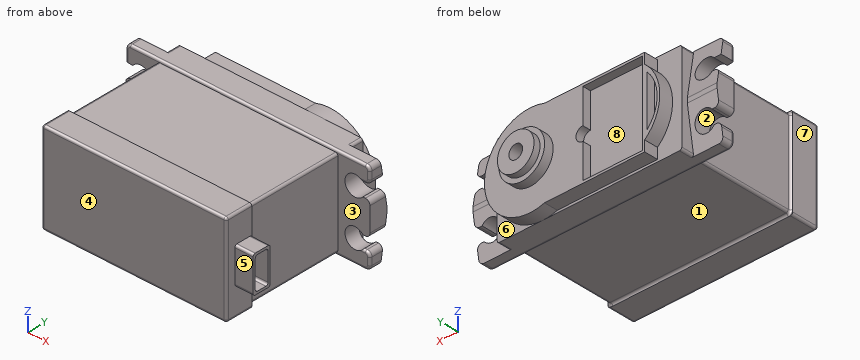
from build123d import *

# Parameters (mm, degrees)
SKETCH_2_W               = 40.3
SKETCH_2_H               = 32
EXTRUDE_1_DEPTH          = 20
SKETCH_3_W               = 20
SKETCH_3_H               = 4
EXTRUDE_2_DEPTH          = 6.5
CUT_EXTRUDE_4_DEPTH      = 6.5
SKETCH_4_W               = 20
SKETCH_4_H               = 4
EXTRUDE_3_DEPTH          = 6.5
CUT_EXTRUDE_5_DEPTH      = 6.5
CUT_EXTRUDE_6_DEPTH      = 43.284026865
CUT_EXTRUDE_6_DEPTH_BACK = 1.5
SKETCH_7_W               = 8
SKETCH_7_H               = 4
SKETCH_7_W_2             = 7
SKETCH_7_H_2             = 3
EXTRUDE_4_DEPTH          = 4
EXTRUDE_5_DEPTH          = 3
SKETCH_9_R               = 5
EXTRUDE_6_DEPTH          = 2
SKETCH_10_R              = 4
EXTRUDE_7_DEPTH          = 1.4
SKETCH_11_R              = 1.5
CUT_EXTRUDE_3_DEPTH      = 6.4
SKETCH_17_W              = 20
SKETCH_17_H              = 20.7
CUT_EXTRUDE_7_DEPTH      = 0.5
SKETCH_18_W              = 39.8
SKETCH_18_H              = 20.7
CUT_EXTRUDE_8_DEPTH      = 0.5
SKETCH_19_W              = 19.5
SKETCH_19_H              = 20.7
CUT_EXTRUDE_9_DEPTH      = 0.5
SKETCH_20_W              = 39.3
SKETCH_20_H              = 20.7
CUT_EXTRUDE_10_DEPTH     = 0.5
FILLET_5_R               = 1
FILLET_6_R               = 0.5
FILLET_7_R               = 0.5
FILLET_8_R               = 0.5
FILLET_9_R               = 0.5
CUT_EXTRUDE_12_DEPTH     = 1.8


with BuildPart() as part:
    # 草圖2 → 填料-伸長1 (new body)
    with BuildSketch(Plane.XY):
        with Locations((2.485695538, -7.217454068)):
            Rectangle(SKETCH_2_W, SKETCH_2_H)
    extrude(amount=EXTRUDE_1_DEPTH)

    # 草圖3 → 填料-伸長2 (add)
    with BuildSketch(Plane(origin=(22.635695538, 0, 0), x_dir=(0, 0, -1), z_dir=(1, 0, 0))):
        with Locations((-10, 5.482545932)):
            Rectangle(SKETCH_3_W, SKETCH_3_H)
    extrude(amount=EXTRUDE_2_DEPTH)

    # 草圖13 → 除料-伸長4 (cut)
    with BuildSketch(Plane(origin=(29.135695538, 0, 0), x_dir=(0, 0, -1), z_dir=(1, 0, 0))):
        Polygon((-20, 5.982545932), (-10.5, 7.482545932), (-20, 7.482545932), align=None)
        Polygon((0, 7.482545932), (-9.5, 7.482545932), (0, 5.982545932), align=None)
    extrude(amount=-CUT_EXTRUDE_4_DEPTH, mode=Mode.SUBTRACT)

    # 草圖4 → 填料-伸長3 (add)
    with BuildSketch(Plane.ZY.offset(17.664304462)):
        with Locations((10, 5.482545932)):
            Rectangle(SKETCH_4_W, SKETCH_4_H)
    extrude(amount=EXTRUDE_3_DEPTH)

    # 草圖14 → 除料-伸長5 (cut)
    with BuildSketch(Plane.ZY.offset(24.164304462)):
        Polygon((0, 5.982545932), (9.5, 7.482545932), (0, 7.482545932), align=None)
        Polygon((20, 7.482545932), (10.5, 7.482545932), (20, 5.982545932), align=None)
    extrude(amount=-CUT_EXTRUDE_5_DEPTH, mode=Mode.SUBTRACT)

    # 草圖16 → 除料-伸長6 (cut, two sides: drawn at the far end of the back side and taken through both)
    with BuildSketch(Plane(origin=(0, 0, 0), x_dir=(1, 0, 0), z_dir=(0, 1, 0)).offset(-CUT_EXTRUDE_6_DEPTH_BACK)):
        with BuildLine():
            Line((-24.164304462, -3.6), (-24.164304462, -6.4))
            Line((-24.164304462, -6.4), (-22.611360737, -6.4))
            ThreePointArc((-22.611360737, -6.4), (-18.714304462, -5), (-22.611360737, -3.6))
            Line((-22.611360737, -3.6), (-24.164304462, -3.6))
        make_face()
        with BuildLine():
            Line((-24.164304462, -13.6), (-24.164304462, -16.4))
            Line((-24.164304462, -16.4), (-22.611360737, -16.4))
            ThreePointArc((-22.611360737, -16.4), (-18.714304462, -15), (-22.611360737, -13.6))
            Line((-22.611360737, -13.6), (-24.164304462, -13.6))
        make_face()
        with BuildLine():
            Line((27.582751813, -16.4), (29.135695538, -16.4))
            Line((29.135695538, -16.4), (29.135695538, -13.6))
            Line((29.135695538, -13.6), (27.582751813, -13.6))
            ThreePointArc((27.582751813, -13.6), (23.685695538, -15), (27.582751813, -16.4))
        make_face()
        with BuildLine():
            Line((27.582751813, -6.4), (29.135695538, -6.4))
            Line((29.135695538, -6.4), (29.135695538, -3.6))
            Line((29.135695538, -3.6), (27.582751813, -3.6))
            ThreePointArc((27.582751813, -3.6), (23.685695538, -5), (27.582751813, -6.4))
        make_face()
    extrude(amount=CUT_EXTRUDE_6_DEPTH + CUT_EXTRUDE_6_DEPTH_BACK, mode=Mode.SUBTRACT)

    # 草圖7 → 填料-伸長4 (add)
    with BuildSketch(Plane(origin=(22.635695538, 0, 0), x_dir=(0, 0, -1), z_dir=(1, 0, 0))):
        with Locations((-10, -19.217454068)):
            Rectangle(SKETCH_7_W, SKETCH_7_H)
        with Locations((-10, -19.217454068)):
            Rectangle(SKETCH_7_W_2, SKETCH_7_H_2, mode=Mode.SUBTRACT)
    extrude(amount=EXTRUDE_4_DEPTH)

    # 草圖8 → 填料-伸長5 (add)
    with BuildSketch(Plane(origin=(0, 8.782545932, 0), x_dir=(1, 0, 0), z_dir=(0, 1, 0))):
        with BuildLine():
            Line((-12.354443672, -17.206398307), (-12.354443672, -19.5))
            Line((-12.354443672, -19.5), (9.513196539, -19.5))
            ThreePointArc((9.513196539, -19.5), (22.635695538, -10), (9.513196539, -0.5))
            Line((9.513196539, -0.5), (-12.354443672, -0.5))
            Line((-12.354443672, -0.5), (-12.354443672, -2.793601693))
            ThreePointArc((-12.354443672, -2.793601693), (-15.664304462, -10), (-12.354443672, -17.206398307))
        make_face()
    extrude(amount=EXTRUDE_5_DEPTH)

    # 草圖9 → 填料-伸長6 (add)
    with BuildSketch(Plane(origin=(0, 11.782545932, 0), x_dir=(1, 0, 0), z_dir=(0, 1, 0))):
        with Locations(Location((12.635695538, -10, 0), (0, 0, 270))):
            Circle(SKETCH_9_R)
    extrude(amount=EXTRUDE_6_DEPTH)

    # 草圖10 → 填料-伸長7 (add)
    with BuildSketch(Plane(origin=(0, 13.782545932, 0), x_dir=(1, 0, 0), z_dir=(0, 1, 0))):
        with Locations(Location((12.635695538, -10, 0), (0, 0, 270))):
            Circle(SKETCH_10_R)
    extrude(amount=EXTRUDE_7_DEPTH)

    # 草圖11 → 除料-伸長3 (cut)
    with BuildSketch(Plane(origin=(0, 15.182545932, 0), x_dir=(1, 0, 0), z_dir=(0, 1, 0))):
        with Locations(Location((12.635695538, -10, 0), (0, 0, 270))):
            Circle(SKETCH_11_R)
    extrude(amount=-CUT_EXTRUDE_3_DEPTH, mode=Mode.SUBTRACT)

    # 草圖17 → 除料-伸長7 (cut)
    with BuildSketch(Plane(origin=(22.635695538, 0, 0), x_dir=(0, 0, -1), z_dir=(1, 0, 0))):
        with Locations((-10, -6.867454068)):
            Rectangle(SKETCH_17_W, SKETCH_17_H)
    extrude(amount=-CUT_EXTRUDE_7_DEPTH, mode=Mode.SUBTRACT)

    # 草圖18 → 除料-伸長8 (cut)
    with BuildSketch(Plane.XY.offset(20)):
        with Locations((2.235695538, -6.867454068)):
            Rectangle(SKETCH_18_W, SKETCH_18_H)
    extrude(amount=-CUT_EXTRUDE_8_DEPTH, mode=Mode.SUBTRACT)

    # 草圖19 → 除料-伸長9 (cut)
    with BuildSketch(Plane.ZY.offset(17.664304462)):
        with Locations((9.75, -6.867454068)):
            Rectangle(SKETCH_19_W, SKETCH_19_H)
    extrude(amount=-CUT_EXTRUDE_9_DEPTH, mode=Mode.SUBTRACT)

    # 草圖20 → 除料-伸長10 (cut)
    with BuildSketch(Plane(origin=(0, 0, 0), x_dir=(-1, 0, 0), z_dir=(0, 0, -1))):
        with Locations((-2.485695538, -6.867454068)):
            Rectangle(SKETCH_20_W, SKETCH_20_H)
    extrude(amount=-CUT_EXTRUDE_10_DEPTH, mode=Mode.SUBTRACT)

    # 圓角5
    fillet_5_edges = [part.edges().sort_by_distance(p)[0] for p in [
        (29.135695538, 5.23780909, 13.6),
        (29.135695538, 5.016756458, 16.4),
        (-24.164304462, 5.23780909, 13.6),
        (29.135695538, 5.016756458, 3.6),
        (29.135695538, 5.23780909, 6.4),
        (-24.164304462, 5.23780909, 6.4),
        (-24.164304462, 5.016756458, 3.6),
        (29.135695538, 4.732545932, 0),
        (29.135695538, 4.732545932, 20),
        (-24.164304462, 4.732545932, 20),
        (-24.164304462, 4.732545932, 0),
    ]]
    fillet(fillet_5_edges, radius=FILLET_5_R)

    # 圓角6
    fillet_6_edges = [part.edges().sort_by_distance(p)[0] for p in [
        (-17.664304462, 7.382545932, 20),
        (22.635695538, -20.217454068, 0),
        (22.635695538, -20.217454068, 20),
        (-17.664304462, -20.217454068, 20),
        (22.135695538, -6.867454068, 19.5),
        (-17.664304462, -20.217454068, 0),
        (-17.164304462, -6.867454068, 19.5),
        (22.135695538, -6.867454068, 0.5),
        (-17.164304462, -6.867454068, 0.5),
        (-17.664304462, 7.382545932, 0),
        (22.635695538, 7.382545932, 0),
        (22.635695538, 7.382545932, 20),
    ]]
    fillet(fillet_6_edges, radius=FILLET_6_R)

    # 圓角7
    fillet_7_edges = [part.edges().sort_by_distance(p)[0] for p in [
        (2.485695538, -23.217454068, 0),
        (22.635695538, -23.217454068, 10),
        (2.485695538, -23.217454068, 20),
        (-17.664304462, -23.217454068, 10),
        (-17.517857853, -23.217454068, 0.146446609),
        (-17.517857853, -23.217454068, 19.853553391),
        (22.489248929, -23.217454068, 19.853553391),
        (22.489248929, -23.217454068, 0.146446609),
        (2.485695538, -17.217454068, 0.5),
        (22.135695538, -17.217454068, 10),
        (2.485695538, -17.217454068, 19.5),
        (-17.164304462, -17.217454068, 10),
        (-17.017857853, -17.217454068, 0.646446609),
        (-17.017857853, -17.217454068, 19.353553391),
        (21.989248929, -17.217454068, 19.353553391),
        (21.989248929, -17.217454068, 0.646446609),
    ]]
    fillet(fillet_7_edges, radius=FILLET_7_R - 0.0001)  # a hair under: the kernel refuses the full size

    # 圓角8
    fillet_8_edges = [part.edges().sort_by_distance(p)[0] for p in [
        (27.859223675, 3.482545932, 3.6),
        (28.842802319, 3.482545932, 3.307106781),
        (29.135695538, 3.482545932, 1.8),
        (28.842802319, 3.482545932, 0.292893219),
        (-22.887832599, 3.482545932, 3.6),
        (-23.871411243, 3.482545932, 3.307106781),
        (-24.164304462, 3.482545932, 1.8),
        (-23.871411243, 3.482545932, 0.292893219),
        (27.859223675, 3.482545932, 16.4),
        (28.842802319, 3.482545932, 16.692893219),
        (29.135695538, 3.482545932, 18.2),
        (28.842802319, 3.482545932, 19.707106781),
        (-24.164304462, 3.482545932, 17.7),
        (-23.871411243, 3.482545932, 19.707106781),
        (2.485695538, 3.482545932, 0),
        (2.485695538, 3.482545932, 20),
    ]]
    fillet(fillet_8_edges, radius=FILLET_8_R - 0.0001)  # a hair under: the kernel refuses the full size

    # 圓角9
    fillet_9_edges = [part.edges().sort_by_distance(p)[0] for p in [
        (24.635695538, -21.217454068, 6),
        (24.635695538, -17.217454068, 6),
        (24.635695538, -17.217454068, 14),
        (24.635695538, -21.217454068, 14),
        (24.635695538, -17.717454068, 6.5),
        (24.635695538, -17.717454068, 13.5),
        (24.635695538, -20.717454068, 13.5),
        (24.635695538, -20.717454068, 6.5),
    ]]
    fillet(fillet_9_edges, radius=FILLET_9_R)

    # 草圖22 → 除料-伸長12 (cut)
    with BuildSketch(Plane(origin=(0, 11.782545932, 0), x_dir=(1, 0, 0), z_dir=(0, 1, 0))):
        with BuildLine():
            Line((1.145556328, -1), (-11.854443672, -1))
            Line((-11.854443672, -1), (-11.854443672, -19))
            Line((-11.854443672, -19), (1.145556328, -19))
            Line((1.145556328, -19), (1.145556328, -11.5))
            ThreePointArc((1.145556328, -11.5), (2.645556328, -10), (1.145556328, -8.5))
            Line((1.145556328, -8.5), (1.145556328, -1))
        make_face()
        with BuildLine():
            Line((-12.854443672, -4.463311785), (-12.854443672, -15.536688215))
            ThreePointArc((-12.854443672, -15.536688215), (-15.079923466, -10), (-12.854443672, -4.463311785))
        make_face()
    extrude(amount=-CUT_EXTRUDE_12_DEPTH, mode=Mode.SUBTRACT)


solid = part.part
For this review, take the finished solid that the model builds, in its own axes (mm). Face numbers are marked on the shaded views. A direction names the side the tool comes from. Round coordinates to 2 decimals unless told otherwise and drop trailing zeros. Order: outer loops, then holes, each group sorted by start corner. A loop starts at its lowest first (then second) coordinate and runs counter-clockwise, first axis right, second up. Notation, with made-up numbers: (-10.5, 28) -> (33.5, 28) arc R16 ccw to (33.5, 57) -> close; hole circle Ø2 at (5, 29.25). An arc over 180 degrees is marked (long way). Put each result on its own line as item: value.
Q1. Insertion check: pin 1 Ø5 at (y, z) = (-16, 17) entering from +X; pin 2 Ø2.5 at (x, y) = (-1, 10.5) entering from +Z; pin 3 Ø2 at (y, z) = (7.5, 14.5) entering from -X. Each pin has a flat end and moves straight along its axis. Give the tip position at first contact, or say it passes through.
Check result:
pin 1: x = 22.64
pin 2: z = 19.5
pin 3: x = -19.18
Q2. Machinability: for the marked faces 5, 6, 7 and 8, which of the approach directions +Z, -Z, +X, -X, +Y, -Y give a long, thin tool a straight path to every point of the face, cutting with its end or side? Answer none if there is none.
Check result:
face 5: +Z, -Z, +X, -Y
face 6: -Z, +X, +Y
face 7: +Z, -Z, -X, -Y
face 8: +Y
Q3. Add section A-A on y = 2.5. Write out the cut boundary in (x, z).
Check result:
outline: (-17.16, 1) arc R0.5 ccw to (-16.66, 0.5) -> (21.64, 0.5) arc R0.5 ccw to (22.14, 1) -> (22.14, 19) arc R0.5 ccw to (21.64, 19.5) -> (-16.66, 19.5) arc R0.5 ccw to (-17.16, 19) -> close
Q4. Add section B-B on x = -21. Write out the cut boundary in (y, z), plus the area to 3 significant figures.
Check result:
outline: (3.48, 0.5) arc R0.5 ccw to (3.98, 0) -> (5.98, 0) -> (6.42, 2.8) -> (3.48, 2.8) -> close; (3.48, 7.2) -> (7.12, 7.2) -> (7.48, 9.5) -> (7.48, 10.5) -> (7.12, 12.8) -> (3.48, 12.8) -> close; (3.48, 17.2) -> (6.42, 17.2) -> (5.98, 20) -> (3.98, 20) arc R0.5 ccw to (3.48, 19.5) -> close
area: 36.7 mm2
Q5. For probe 1 along X at (y, z) = (12.75, 10); probe 2 along Z at (x, y) = (0, 11.5); probe 3 along Y at (x, z) = (18, 12.25), list the stretches that pass through material, from the lowest coordinate up. Write a range as [from, to].
Check result:
probe 1: [7.64, 11.14], [14.14, 17.64]
probe 2: [0.5, 1], [19, 19.5]
probe 3: [-23.22, 11.78]
Q6. Mouldability with a two-part tool opening along Y and no side actions: class the marked faces 1, 2, 3 and 4 as pulls with the +Y half, pulls with the -Y half, needs draft (parallel to the pull), parting line crosses it, or undercut.
Check result:
face 1: undercut
face 2: needs draft
face 3: undercut
face 4: pulls with the -Y half
